from build123d import *

# Parameters (mm, degrees)
SKETCH1_R           = 3.175
BOSS_EXTRUDE1_DEPTH = 3.175


with BuildPart() as part:
    # Sketch1 → Boss-Extrude1 (new body)
    with BuildSketch(Plane(origin=(0, 0, 0), x_dir=(1, 0, 0), z_dir=(0, 1, 0))):
        with BuildLine():
            ThreePointArc((7.9375, 50.8), (0, 58.7375), (-7.9375, 50.8))
            Line((-7.9375, 50.8), (-7.9375, 0))
            ThreePointArc((-7.9375, 0), (0, -7.9375), (7.9375, 0))
            Line((7.9375, 0), (7.9375, 50.8))
        make_face()
        with Locations((0, 50.8)):
            Circle(SKETCH1_R, mode=Mode.SUBTRACT)
        with Locations((0, 25.4)):
            Circle(SKETCH1_R, mode=Mode.SUBTRACT)
        Circle(SKETCH1_R, mode=Mode.SUBTRACT)
    extrude(amount=BOSS_EXTRUDE1_DEPTH)


solid = part.part
Geometry check sheet. Reference: the model listing, model coordinates, mm. Give positions to 0.01 mm unless a question says otherwise; leave off trailing zeros. Write each loop counter-clockwise with the first axis right and the second up, starting at its lowest first coordinate (ties: lowest second). Pieces come first, ordered by that corner, then holes.
1) Cross-section at C-C (z = -23.5). Record the boundary of the cut face in (x, y) (1 decimal), plus the area to 3 significant figures.
Values follow:
outline: (-7.9, 0) - (-2.5, 0) - (-2.5, 3.2) - (-7.9, 3.2) - close; (2.5, 0) - (7.9, 0) - (7.9, 3.2) - (2.5, 3.2) - close
area: 34.3 mm2
2) Cross-section at A-A (x = 0). Record the boundary of the cut face in (y, z) (1 decimal), plus the area to 3 significant figures.
Values follow:
outline: (0, -58.7) - (3.2, -58.7) - (3.2, -54) - (0, -54) - close; (0, -47.6) - (3.2, -47.6) - (3.2, -28.6) - (0, -28.6) - close; (0, -22.2) - (3.2, -22.2) - (3.2, -3.2) - (0, -3.2) - close; (0, 3.2) - (3.2, 3.2) - (3.2, 7.9) - (0, 7.9) - close
area: 151 mm2
3) Thickness scan on line 1 (Z direction, x = 0, y = 1.5) (1 decimal); line 2 (X direction, y = 1.15, z = -25.4) (1 decimal); line 3 (Z direction, x = 1, y = 2.3). Record the ranges inside material, lowest first.
Values follow:
line 1: z = -58.7 to -54, -47.6 to -28.6, -22.2 to -3.2, 3.2 to 7.9
line 2: x = -7.9 to -3.2, 3.2 to 7.9
line 3: z = -58.67 to -53.81, -47.79 to -28.41, -22.39 to -3.01, 3.01 to 7.87
4) Release check for a two-part mould opening along Z. For faces 1 (the face through (0.175, 1.565, -58.736)), 2 (the face through (-0.69, 1.57, 3.1)), 3 (the face through (-0.41, 1.57, -28.55)), 4 (the face through (3.4, 0, -25.9)) record: released by +Z, released by -Z, zero draft, split by the parting line, or undercut.
Values follow:
face 1: released by -Z
face 2: undercut
face 3: undercut
face 4: zero draft
5) Cross-section at B-B (y = 1.35). Count the separate pieces of the cut face and the enclosed holes in it, plus the area to 3 significant figures.
Values follow:
separate pieces: 1
enclosed holes: 3
area: 909 mm2
6) Cross-section at D-D (x = -5.75). Record the boundary of the cut face in (y, z) (3 decimals).
Values follow:
outline: (0, -56.272) - (3.175, -56.272) - (3.175, 5.472) - (0, 5.472) - close
7) Go/stop test with flat-tipped pins: pin 1 Ø1.5 at (x, y) = (-3, 3) entering from -Z; pin 2 Ø7.5 at (x, z) = (0, 0) entering from +Y (3 decimals); pin 3 Ø5.5 at (x, z) = (0, -50.8) entering from +Y. Record where each tip stops, or that it passes through.
Values follow:
pin 1: stops at z = -58.41
pin 2: stops at y = 3.175
pin 3: passes through
